Here's how the part is built. I have some questions about the finished solid (model axes, mm). A direction names the side the tool comes from. Give positions to 0.01 mm unless a question says otherwise; leave off trailing zeros. Loops run counter-clockwise (first coordinate to the right, second up) from the corner with the lowest first, then second, coordinate; pieces in that order, holes last. Notation, with made-up numbers: M 23.5,32.25 L 49.5,32.25 A17 ccw 49.5,49.25 Z; hole C 10,60.5 d6. An arc over 180 degrees is marked long. Answer as CSV lines item,"result". Start each with the question number.
Item 1: I want a section at D-D on x = -19. List the corners of the cut face in (y, z) for me, plus the area to 3 significant figures.
Item 2: I want a section at C-C on z = -1. List the corners of the cut face in (x, y) for me, plus the area to 3 significant figures.
Item 3: If I drill on line 1 along X through (y, z) = (-4.75, 48); line 2 along Z through (x, y) = (-3, -18); line 3 along Y through (x, z) = (34, 27), over which ranges is the centre line in solid material (lowest first)? Write a range as from..to.
Item 4: Will this pin go through, and if not, where does the flat tip stop? P1, Ø5, axis at x = -21, z = 39.5, coming from the -Y side.
Item 5: For faces 5 (the cylindrical face through (-34.928, -10.254, -65.975)), 6 (the cylindrical face through (16.258, -0.913, 38.424)), 7 (the flat face through (0, -1.8, 2)), which set-ups out of +Z, -Z, +X, -X, +Y, -Y let a thin tool reach every point of the face, with its end or its side?
Item 6: If we mould it in two halves opening along X, with no side actions, what happens to faces 1 (the flat face through (-1, -10, -68.982)), 2 (the flat face through (37.47, -10, 0)), 3 (the flat face through (-34.272, -11, 2)), 4 (the cylindrical face through (-34.77, -10.25, 68.15))? For each: released by +X, released by -X, zero draft, split by the parting line, or undercut.
Item 7: I want a section at B-B on x = 5. List the corners of the cut face in (y, z) for me, plus the area to 3 significant figures.
Item 8: I want a section at A-A on y = -12. List the corners of the cut face in (x, z) for me, plus the area to 3 significant figures.
from build123d import *

# Parameters (mm, degrees)
F1_DEPTH = 20.8
F3_DEPTH = 19
F5_DEPTH = 25
F7_DEPTH = 25


with BuildPart() as f1:
    # F0 (on Front) → F1 (new body)
    with BuildSketch(Plane.XZ):
        with BuildLine():
            Line((27.470242, 70.997512), (-27.779758, 70.997512))
            ThreePointArc((-27.779758, 70.997512), (-34.850826, 68.06858), (-37.779758, 60.997512))
            Line((-37.779758, 60.997512), (-37.779758, -58.982488))
            ThreePointArc((-37.779758, -58.982488), (-34.850826, -66.053556), (-27.779758, -68.982488))
            Line((-27.779758, -68.982488), (27.470242, -68.982488))
            ThreePointArc((27.470242, -68.982488), (34.54131, -66.053556), (37.470242, -58.982488))
            Line((37.470242, -58.982488), (37.470242, 60.997512))
            ThreePointArc((37.470242, 60.997512), (34.54131, 68.06858), (27.470242, 70.997512))
        make_face()
    extrude(amount=F1_DEPTH)

    # F2 (on face) → F3 (cut)
    with BuildSketch(Plane.XZ.offset(20.8)):
        with BuildLine():
            Line((24.576889, 68.822538), (-24.272246, 68.822538))
            ThreePointArc((-24.272246, 68.822538), (-31.343314, 65.893605), (-34.272246, 58.822538))
            Line((-34.272246, 58.822538), (-34.272246, -56.564314))
            ThreePointArc((-34.272246, -56.564314), (-31.343314, -63.635382), (-24.272246, -66.564314))
            Line((-24.272246, -66.564314), (24.576889, -66.564314))
            ThreePointArc((24.576889, -66.564314), (31.647957, -63.635382), (34.576889, -56.564314))
            Line((34.576889, -56.564314), (34.576889, 58.822538))
            ThreePointArc((34.576889, 58.822538), (31.647957, 65.893605), (24.576889, 68.822538))
        make_face()
    extrude(amount=-F3_DEPTH, mode=Mode.SUBTRACT)

    # F4 (on face) → F5 (cut)
    with BuildSketch(Plane.XZ.offset(1.8)):
        with BuildLine():
            Line((9.265215, 57.322538), (-2.374785, 57.322538))
            ThreePointArc((-2.374785, 57.322538), (-9.445852, 54.393605), (-12.374785, 47.322538))
            Line((-12.374785, 47.322538), (-12.374785, 21.472538))
            ThreePointArc((-12.374785, 21.472538), (-9.445852, 14.40147), (-2.374785, 11.472538))
            ThreePointArc((-2.374785, 11.472538), (4.696283, 14.40147), (7.625215, 21.472538))
            Line((7.625215, 21.472538), (7.625215, 35.572538))
            Line((7.625215, 35.572538), (9.265215, 35.572538))
            ThreePointArc((9.265215, 35.572538), (16.336283, 38.50147), (19.265215, 45.572538))
            Line((19.265215, 45.572538), (19.265215, 47.322538))
            ThreePointArc((19.265215, 47.322538), (16.336283, 54.393605), (9.265215, 57.322538))
        make_face()
    extrude(amount=-F5_DEPTH, mode=Mode.SUBTRACT)

    # F6 (on face) → F7 (cut)
    with BuildSketch(Plane(origin=(0, 0, 0), x_dir=(-1, 0, 0), z_dir=(0, 1, 0))):
        with BuildLine():
            Line((-11.870242, -47.772488), (-22.780242, -47.772488))
            ThreePointArc((-22.780242, -47.772488), (-23.487349, -48.065381), (-23.780242, -48.772488))
            Line((-23.780242, -48.772488), (-23.780242, -54.292488))
            ThreePointArc((-23.780242, -54.292488), (-23.487349, -54.999594), (-22.780242, -55.292488))
            Line((-22.780242, -55.292488), (-11.870242, -55.292488))
            ThreePointArc((-11.870242, -55.292488), (-11.163135, -54.999594), (-10.870242, -54.292488))
            Line((-10.870242, -54.292488), (-10.870242, -48.772488))
            ThreePointArc((-10.870242, -48.772488), (-11.163135, -48.065381), (-11.870242, -47.772488))
        make_face()
    extrude(amount=-F7_DEPTH, mode=Mode.SUBTRACT)


solid = f1.part
Result:
1,outline,"M -20.8,-68.98 L 0,-68.98 L 0,71 L -20.8,71 L -20.8,68.82 L -1.8,68.82 L -1.8,-66.56 L -20.8,-66.56 Z"
1,area,"339 mm^2"
2,outline,"M -37.78,-20.8 L -34.27,-20.8 L -34.27,-1.8 L 34.58,-1.8 L 34.58,-20.8 L 37.47,-20.8 L 37.47,0 L -37.78,0 Z"
2,area,"257 mm^2"
3,line 1,"-37.78..-34.27, 34.58..37.47"
3,line 2,"-68.98..-66.56, 68.82..71"
3,line 3,"-1.8..0"
4,P1,"y = -1.8"
5,face 5,"-Z, -X, +Y, -Y"
5,face 6,"+Y, -Y"
5,face 7,"-Y"
6,face 1,"zero draft"
6,face 2,"released by +X"
6,face 3,"undercut"
6,face 4,"released by -X"
7,outline,"M -20.8,-68.98 L 0,-68.98 L 0,14.72 L -1.8,14.72 L -1.8,-66.56 L -20.8,-66.56 Z; M -20.8,68.82 L -1.8,68.82 L -1.8,57.32 L 0,57.32 L 0,71 L -20.8,71 Z"
7,area,"263 mm^2"
8,outline,"M -37.78,-58.98 A10 ccw -27.78,-68.98 L 27.47,-68.98 A10 ccw 37.47,-58.98 L 37.47,61 A10 ccw 27.47,71 L -27.78,71 A10 ccw -37.78,61 Z; hole M -34.27,-56.56 A10 ccw -24.27,-66.56 L 24.58,-66.56 A10 ccw 34.58,-56.56 L 34.58,58.82 A10 ccw 24.58,68.82 L -24.27,68.82 A10 ccw -34.27,58.82 Z"
8,area,"1,210 mm^2"
